Input: dimensioned drawing with shaded views. Units: mm. Origin: part minimum x, y, z. A direction names the side the tool comes from. Give positions to 0.01 mm unless a question says otherwise; leave off trailing zeros. Write each loop counter-clockwise with the first axis right and the second up, starting at its lowest first coordinate (ties: lowest second). Pieces come first, ordered by that corner, then holes. Notation, with made-up numbers: (31.25, 43) - (43.25, 43) arc R28 ccw to (43.25, 70) - close; hole circle Ø4 at (87, 16). An arc over 180 degrees is marked (long way). Answer as CSV lines item,"result".
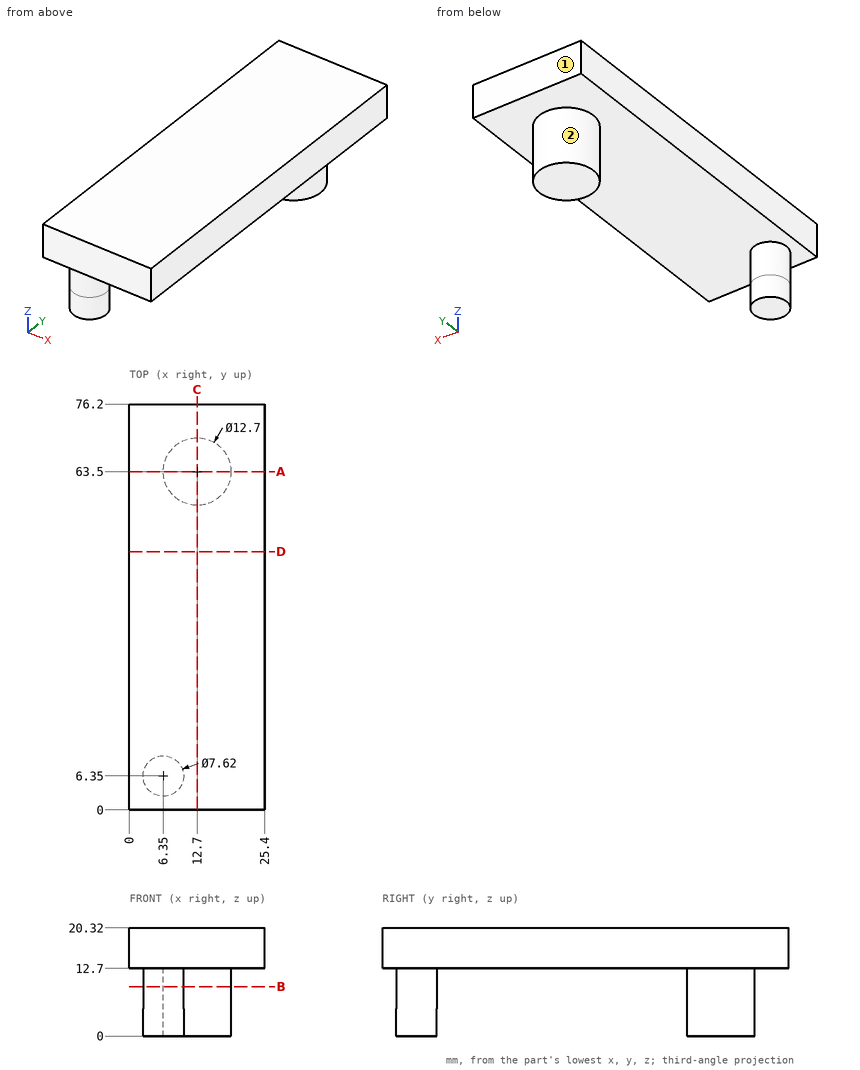
Item 1: Cut plane A-A on y = 63.5. Return the cut outline in (x, z), plus the area to 3 significant figures.
The answers:
outline,"(0, 12.7) - (6.35, 12.7) - (6.35, 0) - (19.05, 0) - (19.05, 12.7) - (25.4, 12.7) - (25.4, 20.32) - (0, 20.32) - close"
area,"355 mm²"
Item 2: Ray query, line 1 (Z direction, x = 14.25, y = 43); line 2 (Y direction, x = 8, z = 10); line 3 (Y direction, x = 8.75, z = 1.25). Return the intervals inside material, ascending. Write a range as from..to.
The answers:
line 1,"12.7..20.32"
line 2,"2.92..9.78, 59.23..67.77"
line 3,"3.39..9.31, 58.53..68.47"
Item 3: Cut plane D-D on y = 48.5. Return the cut outline in (x, z), plus the area to 3 significant figures.
The answers:
outline,"(0, 12.7) - (25.4, 12.7) - (25.4, 20.32) - (0, 20.32) - close"
area,"194 mm²"
Item 4: Cut plane C-C on x = 12.7. Return the cut outline in (y, z), plus the area to 3 significant figures.
The answers:
outline,"(0, 12.7) - (57.15, 12.7) - (57.15, 0) - (69.85, 0) - (69.85, 12.7) - (76.2, 12.7) - (76.2, 20.32) - (0, 20.32) - close"
area,"742 mm²"
Item 5: Reachability of the marked faces 1 and 2 from +Z, -Z, +X, -X, +Y, -Y: full face, straight path, thin tool, end or side. Return the list, or none.
The answers:
face 1,"+Z, -Z, +X, -X, +Y"
face 2,"-Z"
Item 6: Contact query for a flat-ended pin moving along its axis: pin 1 (6 mm diameter, centred on x = 8.5, y = 51, fed in from -Z). Output: stop coordinate, or through.
The answers:
pin 1,"z = 12.7"
Item 7: Cut plane B-B on z = 9.25. Return the cut outline in (x, y), plus the area to 3 significant figures.
The answers:
outline,"circle Ø7.62 at (6.35, 6.35); circle Ø12.7 at (12.7, 63.5)"
area,"172 mm²"
